from build123d import *

# Parameters (mm, degrees)
SKETCH1_R           = 5
BOSS_EXTRUDE1_DEPTH = 18.5
SKETCH2_R           = 2
CUT_EXTRUDE1_DEPTH  = 18.5
SKETCH3_R           = 3.65
CUT_EXTRUDE2_DEPTH  = 3.5
CUT_EXTRUDE3_START  = -10.5
SKETCH4_R           = 3.65
CUT_EXTRUDE3_DEPTH  = 10.5
CHAMFER1_SIZE       = 1.5
CHAMFER2_SIZE       = 1
CUT_EXTRUDE4_DEPTH  = 5


with BuildPart() as part:
    # Sketch1 → Boss-Extrude1 (new body)
    with BuildSketch(Plane.XY):
        Circle(SKETCH1_R)
    extrude(amount=BOSS_EXTRUDE1_DEPTH)

    # Sketch2 → Cut-Extrude1 (cut)
    with BuildSketch(Plane.XY.offset(18.5)):
        Circle(SKETCH2_R)
    extrude(amount=-CUT_EXTRUDE1_DEPTH, mode=Mode.SUBTRACT)

    # Sketch3 → Cut-Extrude2 (cut)
    with BuildSketch(Plane.XY.offset(18.5)):
        Circle(SKETCH3_R)
    extrude(amount=-CUT_EXTRUDE2_DEPTH, mode=Mode.SUBTRACT)

    # Sketch4 → Cut-Extrude3 (cut)
    with BuildSketch(Plane(origin=(0, 0, 0), x_dir=(-1, 0, 0), z_dir=(0, 0, -1)).offset(CUT_EXTRUDE3_START)):
        with Locations(Location((0, 0, 0), (0, 0, 180))):
            Circle(SKETCH4_R)
    extrude(amount=CUT_EXTRUDE3_DEPTH, mode=Mode.SUBTRACT)

    # Chamfer1
    chamfer1_edges = [part.edges().sort_by_distance(p)[0] for p in [
        (-2, 0, 10.5),
    ]]
    chamfer(chamfer1_edges, length=CHAMFER1_SIZE)

    # Chamfer2
    chamfer2_edges = [part.edges().sort_by_distance(p)[0] for p in [
        (-2, 0, 15),
    ]]
    chamfer(chamfer2_edges, length=CHAMFER2_SIZE)

    # Sketch5 → Cut-Extrude4 (cut)
    with BuildSketch(Plane(origin=(0, 0, 0), x_dir=(-1, 0, 0), z_dir=(0, 0, -1))):
        Polygon((0, 4.214656965), (-3.65, 2.107328483), (-3.65, -2.107328483), (0, -4.214656965), (3.65, -2.107328483), (3.65, 2.107328483), align=None)
    extrude(amount=-CUT_EXTRUDE4_DEPTH, mode=Mode.SUBTRACT)


solid = part.part
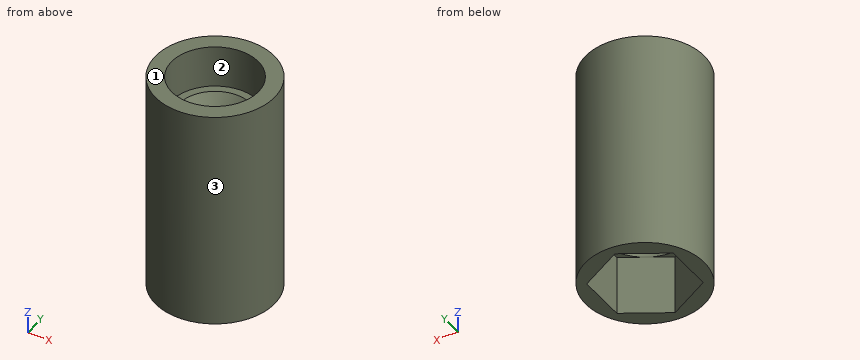
Design review of the part built by this model. Coordinates are the model's own, in mm. Face numbers are marked on the shaded views. Round coordinates to 2 decimals unless told otherwise and drop trailing zeros. Write each loop counter-clockwise with the first axis right and the second up, starting at its lowest first coordinate (ties: lowest second). Pieces come first, ordered by that corner, then holes. Notation, with made-up numbers: M 69.25,37 L 116.25,37 A19 ccw 116.25,42 Z; hole C 64.25,22.25 d6. An arc over 180 degrees is marked long. One line per item, written item: value. Start each with the question number.
1. Take a section at B-B on z = 5.5. State the section outline as (x, y) points.
2. Take a section at C-C on z = 13.75. State the section outline as (x, y) points, then the cut area to 3 significant figures.
3. To check wall thickness, follow probe 1 along Y at (x, z) = (0, 6.6); probe 2 along Y at (x, z) = (0, 13.3); probe 3 along X at (y, z) = (-3.25, 8.75). State the ranges of each line that lie inside material, in increasing order. Write a range as from..to.
4. Draft analysis for pull direction Y (two halves, no side actions). For the marked faces 1, 2 and 3, state which applies: pulls with the +Y half, pulls with the -Y half, needs draft (parallel to the pull), parting line crosses it, or undercut.
5. Clearance check with flat-ended pins moving along their axes: P1, Ø1, axis at y = -4, z = 13.5, coming from the +X side; P2, Ø1, axis at y = -2, z = 7.5, coming from the -X side; P3, Ø1.5, axis at x = -3, z = 14.5, coming from the -Y side. State where each tip first meets the part, or that it passes through.
6. Take a section at A-A on z = 2. State the section outline as (x, y) points.
Computed:
1. outline: C 0,0 d10; hole C 0,0 d7.3
2. outline: C 0,0 d10; hole C 0,0 d4
2. area: 66.0 mm²
3. probe 1: y = -5..-3.65, 3.65..5
3. probe 2: y = -5..-2, 2..5
3. probe 3: x = -3.8..-1.66, 1.66..3.8
4. face 1: needs draft
4. face 2: undercut
4. face 3: parting line crosses it
5. P1: stops at x = 3.57
5. P2: stops at x = -4.77
5. P3: stops at y = -4.47
6. outline: C 0,0 d10; hole M -3.65,-2.11 L 0,-4.21 L 3.65,-2.11 L 3.65,2.11 L 0,4.21 L -3.65,2.11 Z
